The model under review builds one solid part; all positions refer to its coordinate system, in mm. Round coordinates to 2 decimals unless told otherwise and drop trailing zeros. Loops run counter-clockwise (first coordinate to the right, second up) from the corner with the lowest first, then second, coordinate; pieces in that order, holes last. Notation, with made-up numbers: M 27,57.25 L 55,57.25 A21 ccw 55,70.25 Z; hole C 65,31 d1. An arc over 180 degrees is marked long. Answer as a JSON object with one key per item and string values. Group by question number.
Item 1: To check wall thickness, follow line 1 (X direction, y = -14, z = 1); line 2 (Y direction, x = 9.25, z = 3.7); line 3 (Y direction, x = -7, z = 0.3). State the ranges of each line that lie inside material, in increasing order.
Item 2: Consider section B-B (z = 2.95). Give the boundary of the cut face in (x, y).
Item 3: Consider section C-C (y = 35). Give the boundary of the cut face in (x, z).
Item 4: Consider section A-A (x = -7.75). Give the boundary of the cut face in (y, z), and give its area (3 significant figures).
```python
from build123d import *

# Parameters (mm, degrees)
F1_DEPTH = 4


with BuildPart() as f1:
    # F0 (on Top) → F1 (new body)
    with BuildSketch(Plane.XY):
        with BuildLine():
            Line((-5, 40), (-5, 0))
            Line((-5, 0), (0, 0))
            Line((0, 0), (0, 84.662878))
            Line((0, 84.662878), (-10, 84.662878))
            Line((-10, 84.662878), (-10, 54.662878))
            ThreePointArc((-10, 54.662878), (-6.284367, 47.745967), (-5, 40))
        make_face()
    extrude(amount=F1_DEPTH)

    # F2: F1 across face


with BuildPart() as f1_1:
    add(f1.part)
    add(f1.part.mirror(Plane(origin=(0, 42.331439, 2), x_dir=(0, 1, 0), z_dir=(1, 0, 0))))

    # F3: F1 across face


with BuildPart() as f1_2:
    add(f1_1.part)
    add(f1_1.part.mirror(Plane(origin=(0, 0, 2), x_dir=(1, 0, 0), z_dir=(0, -1, 0))))


solid = f1_2.part
```
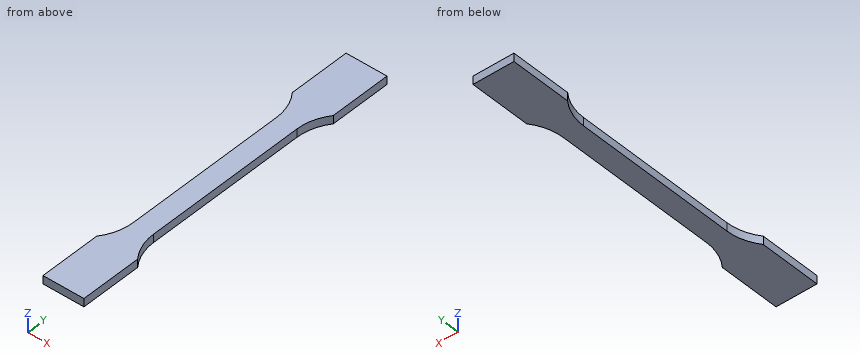
Geometry results:
{
 "1": {"line 1": "x = -5 to 5", "line 2": "y = -84.66 to -53.64, 53.64 to 84.66", "line 3": "y = -84.66 to -49.59, 49.59 to 84.66"},
 "2": {"outline": "M -10,-84.66 L 10,-84.66 L 10,-54.66 A24 cw 5,-40 L 5,40 A24 cw 10,54.66 L 10,84.66 L -10,84.66 L -10,54.66 A24 cw -5,40 L -5,-40 A24 cw -10,-54.66 Z"},
 "3": {"outline": "M -5,0 L 5,0 L 5,4 L -5,4 Z"},
 "4": {"outline": "M -84.66,0 L -51.16,0 L -51.16,4 L -84.66,4 Z; M 51.16,0 L 84.66,0 L 84.66,4 L 51.16,4 Z", "area": "268 mm^2"}
}
